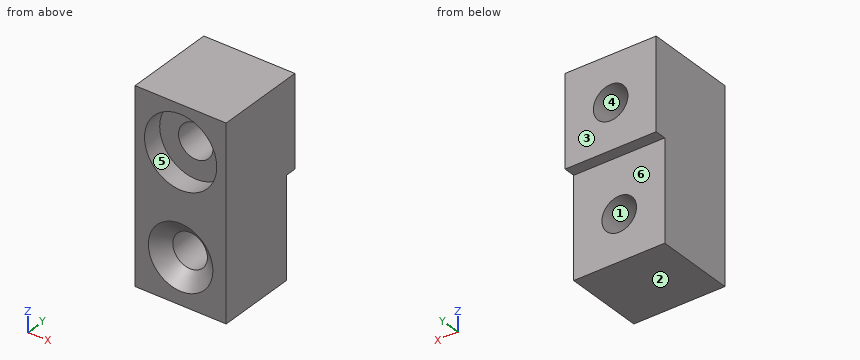
```python
from build123d import *

# Parameters (mm, degrees)
SKETCH1_W                                           = 10
SKETCH1_H                                           = 21
BOSS_EXTRUDE1_DEPTH                                 = 10
SKETCH2_W                                           = 10
SKETCH2_H                                           = 11
CUT_EXTRUDE1_DEPTH                                  = 1.25
CBORE_FOR_6_BINDING_HEAD_MACHINE_SCREW1_D           = 3.7973
CBORE_FOR_6_BINDING_HEAD_MACHINE_SCREW1_CBORE_D     = 7.9375
CBORE_FOR_6_BINDING_HEAD_MACHINE_SCREW1_CBORE_DEPTH = 2.2098
CSK_FOR_6_FLAT_HEAD_MACHINE_SCREW_100_D             = 3.7973
CSK_FOR_6_FLAT_HEAD_MACHINE_SCREW_100_CSINK_D       = 7.0866
CSK_FOR_6_FLAT_HEAD_MACHINE_SCREW_100_CSINK_ANGLE   = 100


with BuildPart() as part:
    # Sketch1 → Boss-Extrude1 (new body)
    with BuildSketch(Plane(origin=(0, 0, 0), x_dir=(1, 0, 0), z_dir=(0, 1, 0))):
        Rectangle(SKETCH1_W, SKETCH1_H)
    extrude(amount=BOSS_EXTRUDE1_DEPTH)

    # Sketch2 → Cut-Extrude1 (cut)
    with BuildSketch(Plane(origin=(0, 10, 0), x_dir=(1, 0, 0), z_dir=(0, 1, 0))):
        with Locations((0, 5)):
            Rectangle(SKETCH2_W, SKETCH2_H)
    extrude(amount=-CUT_EXTRUDE1_DEPTH, mode=Mode.SUBTRACT)

    # CBORE for #6 Binding Head Machine Screw1 (through all)
    with Locations(Plane(origin=(0, 0, 0), x_dir=(-1, 0, 0), z_dir=(0, -1, 0))):
        with Locations((0, -5.5)):
            CounterBoreHole(CBORE_FOR_6_BINDING_HEAD_MACHINE_SCREW1_D / 2, CBORE_FOR_6_BINDING_HEAD_MACHINE_SCREW1_CBORE_D / 2, CBORE_FOR_6_BINDING_HEAD_MACHINE_SCREW1_CBORE_DEPTH)

    # CSK for #6 Flat Head Machine Screw (100)1 (through all)
    with Locations(Plane(origin=(0, 0, 0), x_dir=(-1, 0, 0), z_dir=(0, -1, 0))):
        with Locations((0, 5.5)):
            CounterSinkHole(CSK_FOR_6_FLAT_HEAD_MACHINE_SCREW_100_D / 2, CSK_FOR_6_FLAT_HEAD_MACHINE_SCREW_100_CSINK_D / 2, counter_sink_angle=CSK_FOR_6_FLAT_HEAD_MACHINE_SCREW_100_CSINK_ANGLE)


solid = part.part
```
Source: CAD feature listing. Evaluate the final solid. Frame: model axes, mm. Face numbers are marked on the shaded views. A direction names the side the tool comes from. Round coordinates to 2 decimals unless told otherwise and drop trailing zeros. Loops run counter-clockwise (first coordinate to the right, second up) from the corner with the lowest first, then second, coordinate; pieces in that order, holes last. Notation, with made-up numbers: M 55.25,-24.75 L 74.25,-24.75 A27 cw 74.25,7.25 Z; hole C -7.75,53.5 d8. An arc over 180 degrees is marked long. Use a Markdown table: item, result. Add a question column.
1. Line query: line 1 (Z direction, x = 0, y = 6.75); line 2 (Z direction, x = 1.25, y = 8); line 3 (Y direction, x = 4.75, z = -7). Output: solid intervals per line, ascending.
2. Section query D-D on z = 5.5. Return the cut outline in (x, y).
3. Reachability of the marked faces 4, 5 and 6 from +Z, -Z, +X, -X, +Y, -Y: full face, straight path, thin tool, end or side. Return the list, or none.
4. Contact query for flat-ended pins moving along their axis: P1, Ø5, axis at x = 0.5, z = -4, coming from the +Y side; P2, Ø2, axis at x = -1.5, z = -7, coming from the -Y side; P3, Ø2.5, axis at x = 0, z = 5.5, coming from the -Y side; P4, Ø2.5, axis at x = -1.5, z = 6.5, coming from the -Y side. Output: stop coordinate, or through.
5. Section query C-C on y = 2. Return the cut outline in (x, z), then the cut area to 3 significant figures.
6. Section query A-A on z = -5.5. Return the cut outline in (x, y).
7. Section query B-B on x = 0. Return the cut outline in (y, z), then the cut area to 3 significant figures.
8. Mould query, pull axis Z, two halves, no side actions, for the marked faces 1, 2 and 3. Classes: pulls with the +Z half, pulls with the -Z half, needs draft (parallel to the pull), parting line crosses it, or undercut.
Reported:
| question | item | result |
|---|---|---|
| 1 | line 1 | z = -10.5 to -7.4, -3.6 to 3.6, 7.4 to 10.5 |
| 1 | line 2 | z = -10.5 to -6.93, -4.07 to 4.07, 6.93 to 10.5 |
| 1 | line 3 | y = 0 to 8.75 |
| 2 | outline | M -5,0 L -3.97,0 L -3.97,2.21 L -1.9,2.21 L -1.9,10 L -5,10 Z; M 1.9,2.21 L 3.97,2.21 L 3.97,0 L 5,0 L 5,10 L 1.9,10 Z |
| 3 | face 4 | +Y, -Y |
| 3 | face 5 | -Y |
| 3 | face 6 | -Z, +X, -X, +Y |
| 4 | P1 | stops at y = 8.75 |
| 4 | P2 | stops at y = 0.35 |
| 4 | P3 | passes through |
| 4 | P4 | stops at y = 2.21 |
| 5 | outline | M -5,-10.5 L 5,-10.5 L 5,10.5 L -5,10.5 Z; hole C 0,5.5 d7.94; hole C 0,-5.5 d3.8 |
| 5 | area | 149 mm² |
| 6 | outline | M -5,0 L -3.54,0 L -1.9,1.38 L -1.9,8.75 L -5,8.75 Z; M 1.9,1.38 L 3.54,0 L 5,0 L 5,8.75 L 1.9,8.75 Z |
| 7 | outline | M 0,-10.5 L 8.75,-10.5 L 8.75,-7.4 L 1.38,-7.4 L 0,-9.04 Z; M 0,-1.96 L 1.38,-3.6 L 8.75,-3.6 L 8.75,0.5 L 10,0.5 L 10,3.6 L 2.21,3.6 L 2.21,1.53 L 0,1.53 Z; M 0,9.47 L 2.21,9.47 L 2.21,7.4 L 10,7.4 L 10,10.5 L 0,10.5 Z |
| 7 | area | 114 mm² |
| 8 | face 1 | undercut |
| 8 | face 2 | pulls with the -Z half |
| 8 | face 3 | needs draft |
